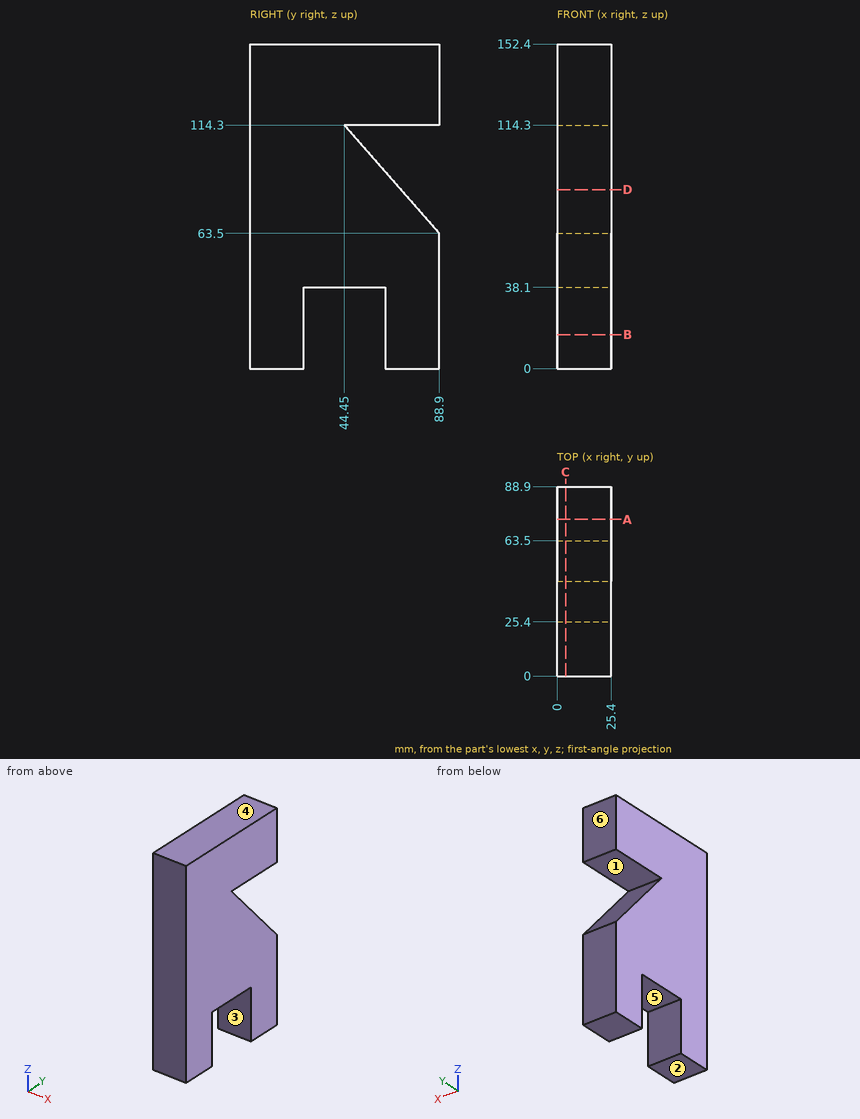
Source: three-view drawing plus pictorial views. Frame: mm from the lowest corner of the part. A direction names the side the tool comes from. Coordinates: 2 decimals unless noted, no trailing zeros. Order: outer loops, then holes, each group sorted by start corner. A loop starts at its lowest first (then second) coordinate and runs counter-clockwise, first axis right, second up. Notation, with made-up numbers: M 44.5,-24.75 L 71.5,-24.75 A20 cw 71.5,3.25 Z; hole C 77,87.25 d8. An arc over 180 degrees is marked long. One line per question, with ' | ' between items.
Item 1: Draft query along Z for the marked faces 1, 2, 3 and 4. Return one class per face: released by +Z, released by -Z, zero draft, split by the parting line, or undercut.
Geometry results:
face 1: undercut | face 2: released by -Z | face 3: zero draft | face 4: released by +Z
Item 2: Section C-C (x = 4). Output: boundary loops of the cut face in (y, z).
Geometry results:
outline: M 0,0 L 25.4,0 L 25.4,38.1 L 63.5,38.1 L 63.5,0 L 88.9,0 L 88.9,63.5 L 44.45,114.3 L 88.9,114.3 L 88.9,152.4 L 0,152.4 Z
Item 3: Section D-D (z = 84). Output: boundary loops of the cut face in (x, y).
Geometry results:
outline: M 0,0 L 25.4,0 L 25.4,70.96 L 0,70.96 Z
Item 4: Ray query, line 1 along Y through (x, z) = (17, 15); line 2 along Z through (x, y) = (22.25, 32.5); line 3 along Z through (x, y) = (23.5, 70). Return the intervals inside material, ascending.
Geometry results:
line 1: y = 0 to 25.4, 63.5 to 88.9 | line 2: z = 38.1 to 152.4 | line 3: z = 0 to 85.1, 114.3 to 152.4
Item 5: Pin query (flat end, axial travel): pin 1 (7.5 mm diameter, centred on x = 12, y = 58, fed in from -Z). Return the tip coordinate at first contact, or that it passes through.
Geometry results:
pin 1: stops at z = 38.1
Item 6: Section B-B (z = 16). Output: boundary loops of the cut face in (x, y).
Geometry results:
outline: M 0,0 L 25.4,0 L 25.4,25.4 L 0,25.4 Z; M 0,63.5 L 25.4,63.5 L 25.4,88.9 L 0,88.9 Z
Item 7: Reachability of the marked faces 5 and 6 from +Z, -Z, +X, -X, +Y, -Y: full face, straight path, thin tool, end or side. Return the list, or none.
Geometry results:
face 5: -Z, +X, -X | face 6: +Z, -Z, +X, -X, +Y
Item 8: Section A-A (y = 73.5). Output: boundary loops of the cut face in (x, z).
Geometry results:
outline: M 0,0 L 25.4,0 L 25.4,81.1 L 0,81.1 Z; M 0,114.3 L 25.4,114.3 L 25.4,152.4 L 0,152.4 Z
